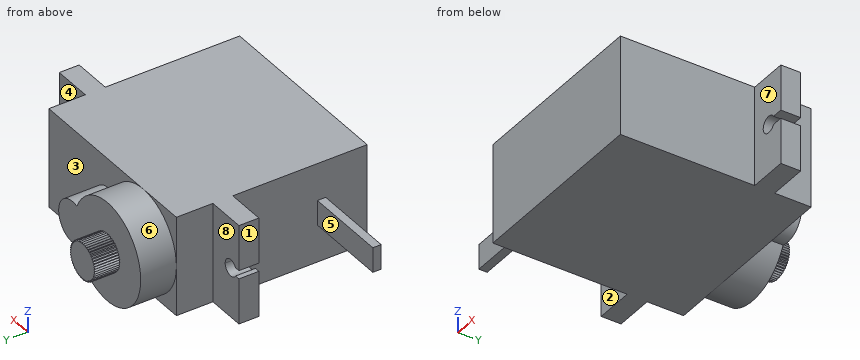
```python
from build123d import *

# Parameters (mm, degrees)
SKETCH2_W           = 23
SKETCH2_H           = 12
BOSS_EXTRUDE1_DEPTH = 23
BOSS_EXTRUDE2_START = -4.4
BOSS_EXTRUDE2_DEPTH = 2.4
SKETCH4_R           = 6
SKETCH4_R_2         = 2.5
BOSS_EXTRUDE3_DEPTH = 4.3
BOSS_EXTRUDE4_DEPTH = 3
SKETCH6_W           = 3
SKETCH6_H           = 1
BOSS_EXTRUDE5_DEPTH = 10


with BuildPart() as part:
    # Sketch2 → Boss-Extrude1 (new body)
    with BuildSketch(Plane(origin=(0, 0, 0), x_dir=(1, 0, 0), z_dir=(0, 1, 0))):
        Rectangle(SKETCH2_W, SKETCH2_H)
    extrude(amount=-BOSS_EXTRUDE1_DEPTH)

    # Sketch3 → Boss-Extrude2 (add)
    with BuildSketch(Plane(origin=(0, 0, 0), x_dir=(1, 0, 0), z_dir=(0, 1, 0)).offset(BOSS_EXTRUDE2_START)):
        with BuildLine():
            Line((-16.2, -0.5), (-16.2, -6))
            Line((-16.2, -6), (-11.5, -6))
            Line((-11.5, -6), (-11.5, 6))
            Line((-11.5, 6), (-16.2, 6))
            Line((-16.2, 6), (-16.2, 0.5))
            Line((-16.2, 0.5), (-15.584293743, 0.5))
            ThreePointArc((-15.584293743, 0.5), (-14.459449294, 0.965925826), (-13.718268339, 0))
            ThreePointArc((-13.718268339, 0), (-14.459449294, -0.965925826), (-15.584293743, -0.5))
            Line((-15.584293743, -0.5), (-16.2, -0.5))
        make_face()
        with BuildLine():
            Line((11.5, 6), (11.5, -6))
            Line((11.5, -6), (16.2, -6))
            Line((16.2, -6), (16.2, -0.5))
            Line((16.2, -0.5), (14.894380034, -0.5))
            ThreePointArc((14.894380034, -0.5), (13.02835463, 0), (14.894380034, 0.5))
            Line((14.894380034, 0.5), (16.2, 0.5))
            Line((16.2, 0.5), (16.2, 6))
            Line((16.2, 6), (11.5, 6))
        make_face()
    extrude(amount=-BOSS_EXTRUDE2_DEPTH)

    # Sketch4 → Boss-Extrude3 (add)
    with BuildSketch(Plane(origin=(0, 0, 0), x_dir=(1, 0, 0), z_dir=(0, 1, 0))):
        with Locations((-5.5, 0)):
            Circle(SKETCH4_R)
        with Locations((0.8, 0)):
            Circle(SKETCH4_R_2)
    extrude(amount=BOSS_EXTRUDE3_DEPTH)

    # Sketch5 → Boss-Extrude4 (add)
    with BuildSketch(Plane(origin=(0, 4.3, 0), x_dir=(1, 0, 0), z_dir=(0, 1, 0))):
        Polygon((-3.255005568, -0.15), (-3.437184296, 0), (-3.255005568, 0.15), (-3.455589794, 0.274946425), (-3.295142762, 0.44844683), (-3.51047784, 0.544986424), (-3.374587739, 0.738324266), (-3.600868956, 0.805301127), (-3.491960749, 1.015026288), (-3.725150111, 1.051245213), (-3.645167266, 1.273615142), (-3.881103504, 1.278429803), (-3.831473318, 1.509476304), (-4.065946143, 1.482800783), (-4.047554268, 1.718400825), (-4.276379508, 1.660711148), (-4.289554146, 1.896660443), (-4.508648409, 1.808986083), (-4.553154459, 2.04107411), (-4.758608002, 1.924979619), (-4.833651254, 2.149064761), (-5.021797754, 2.006621847), (-5.126039057, 2.218705301), (-5.293521035, 2.052455862), (-5.425100203, 2.248752992), (-5.568928939, 2.061663752), (-5.725497937, 2.238671633), (-5.843106805, 2.034081205), (-6.021871655, 2.188641125), (-6.111161921, 1.97020043), (-6.308932561, 2.099554265), (-6.368310838, 1.871161381), (-6.581558046, 1.973000809), (-6.609964728, 1.738731414), (-6.834883102, 1.811239107), (-6.831811271, 1.575273743), (-7.064387138, 1.6171558), (-7.02989161, 1.383705275), (-7.265974648, 1.39421431), (-7.200670997, 1.167444554), (-7.436048299, 1.146393032), (-7.34110187, 0.930350756), (-7.571573122, 0.878114343), (-7.448678237, 0.676654828), (-7.670130674, 0.594165683), (-7.521480394, 0.410883978), (-7.729962192, 0.299614123), (-7.558209186, 0.137780894), (-7.749999982, -0.000284059), (-7.558209186, -0.137780894), (-7.729886469, -0.300177172), (-7.521480394, -0.410883978), (-7.669980579, -0.594713616), (-7.448678237, -0.676654828), (-7.571351335, -0.878637381), (-7.34110187, -0.930350756), (-7.435758777, -1.146881842), (-7.200670997, -1.167444554), (-7.265622557, -1.394660168), (-7.02989161, -1.383705275), (-7.063978761, -1.617550752), (-6.831811271, -1.575273743), (-6.834425728, -1.811576103), (-6.609964728, -1.738731414), (-6.581059835, -1.973273836), (-6.368310838, -1.871161381), (-6.308402404, -2.099758451), (-6.111161921, -1.97020043), (-6.021319013, -2.188772827), (-5.843106805, -2.034081205), (-5.724932672, -2.238728499), (-5.568928939, -2.061663752), (-5.424532402, -2.248734009), (-5.293521035, -2.052455862), (-5.125478853, -2.218610806), (-5.021797754, -2.006621847), (-4.833108643, -2.148896442), (-4.758608002, -1.924979619), (-4.552639125, -2.040834969), (-4.508648409, -1.808986083), (-4.289075284, -1.896354748), (-4.276379508, -1.660711148), (-4.047120423, -1.718034032), (-4.065946143, -1.482800783), (-3.831092233, -1.509054958), (-3.881103504, -1.278429803), (-3.644845742, -1.273146762), (-3.725150111, -1.051245213), (-3.491704522, -1.014519232), (-3.600868956, -0.805301127), (-3.374401382, -0.737787582), (-3.51047784, -0.544986424), (-3.295029601, -0.447890096), (-3.455589794, -0.274946425), align=None)
    extrude(amount=BOSS_EXTRUDE4_DEPTH)

    # Sketch6 → Boss-Extrude5 (add)
    with BuildSketch(Plane.ZY.offset(11.5)):
        with Locations((0, -17.5)):
            Rectangle(SKETCH6_W, SKETCH6_H)
    extrude(amount=BOSS_EXTRUDE5_DEPTH)


solid = part.part
```
Here's how the part is built. I have some questions about the finished solid (model axes, mm). Face numbers are marked on the shaded views. A direction names the side the tool comes from. Coordinates: 2 decimals unless noted, no trailing zeros. Loops run counter-clockwise (first coordinate to the right, second up) from the corner with the lowest first, then second, coordinate; pieces in that order, holes last. Notation, with made-up numbers: M 80,70.5 L 127,70.5 A22 cw 127,85.5 Z; hole C 48.5,-15.5 d5. An arc over 180 degrees is marked long. One line per item, written item: value.
1. On a 3-axis mill with a long thin cutter (end or side, diameter ignored), from which of +Z, -Z, +X, -X, +Y, -Y can I reach the whole of each face in a straight line? I mean the marked faces 4, 5, 6, 7 and 8. Say none if no direction works.
Geometry says:
face 4: +Z, -Z, +X, +Y
face 5: +Z, -Z, -X
face 6: +Y
face 7: +Z, -Z, +X, -Y
face 8: +Z, -Z, -X, +Y
2. Imagine slicing it at D-D (z = 4). List the corners of the cut face in (x, y) for me, and give its area (3 significant figures).
Geometry says:
outline: M -16.2,-6.8 L -11.5,-6.8 L -11.5,-23 L 11.5,-23 L 11.5,-6.8 L 16.2,-6.8 L 16.2,-4.4 L 11.5,-4.4 L 11.5,0 L -1.03,0 L -1.03,4.3 L -9.97,4.3 L -9.97,0 L -11.5,0 L -11.5,-4.4 L -16.2,-4.4 Z
area: 590 mm2
3. Imagine slicing it at B-B (y = -6). List the corners of the cut face in (x, z) for me.
Geometry says:
outline: M -16.2,-6 L 16.2,-6 L 16.2,-0.5 L 14.89,-0.5 A1 cw long 14.89,0.5 L 16.2,0.5 L 16.2,6 L -16.2,6 L -16.2,0.5 L -15.58,0.5 A1 cw long -15.58,-0.5 L -16.2,-0.5 Z
4. Imagine slicing it at C-C (x = 0.8). List the corners of the cut face in (y, z) for me, and give its area (4 significant figures).
Geometry says:
outline: M -23,-6 L 0,-6 L 0,-2.5 L 4.3,-2.5 L 4.3,2.5 L 0,2.5 L 0,6 L -23,6 Z
area: 297.5 mm2
5. Thinking about a two-plate mould opening in Y: for the marked faces 1, 2 and 3, which applies, +Y half, -Y half, draft (parallel to the pull), parting line (faces both ways), or undercut?
Geometry says:
face 1: draft
face 2: undercut
face 3: +Y half
6. Imagine slicing it at A-A (x = -12). List the corners of the cut face in (y, z) for me, and give its area (3 significant figures).
Geometry says:
outline: M -18,-1.5 L -17,-1.5 L -17,1.5 L -18,1.5 Z; M -6.8,-6 L -4.4,-6 L -4.4,6 L -6.8,6 Z
area: 31.8 mm2
7. Will these pins go through, and if not, where does the flat tip stop? pin 1 Ø2.5 at (x, z) = (-14, 1.5) entering from -Y; pin 2 Ø3.5 at (y, z) = (-1.5, 0) entering from +X; pin 3 Ø1.5 at (y, z) = (-12.5, 2.5) entering from -X; pin 4 Ø2 at (x, y) = (-16, -7.5) entering from -Z.
Geometry says:
pin 1: stops at y = -18
pin 2: stops at x = 11.5
pin 3: stops at x = -11.5
pin 4: stops at z = -6
8. Please list where these lines run through material, in increasing order: probe 1 along Y at (x, z) = (-16, -1); probe 2 along Y at (x, z) = (9.5, -5.5); probe 3 along Y at (x, z) = (-16, -2.75).
Geometry says:
probe 1: y = -18 to -17, -6.8 to -4.4
probe 2: y = -23 to 0
probe 3: y = -6.8 to -4.4
